Check sheet for the drawn part. Datum: minimum x, y, z corner. Units: mm. Give positions to 0.01 mm unless a question says otherwise; leave off trailing zeros. Loops run counter-clockwise (first coordinate to the right, second up) from the corner with the lowest first, then second, coordinate; pieces in that order, holes last. Notation, with made-up numbers: (20, 68) - (34, 68) arc R29 ccw to (34, 95) - close; hole circle Ø7 at (-16, 18.25). An arc over 180 degrees is marked (long way). One line per item, written item: value. Start each with the question number.
1. Sectioned sample at B-B (y = 39.5). Record the cut outline in (x, z), plus the area to 3 significant figures.
2. Sectioned sample at A-A (z = 7.5). Record the cut outline in (x, y).
3. Gauge pin test, flat end, axial feed: pin 1 (7.5 mm diameter, centred on y = 38.5, z = 8.5, fed in from -X). Record the tip position at first contact, or that the pin passes through.
4. Scan line: L1, parallel to X at y = 12.5, z = 6.25. Record every from-to range of solid material in increasing order. Write a range as [from, to].
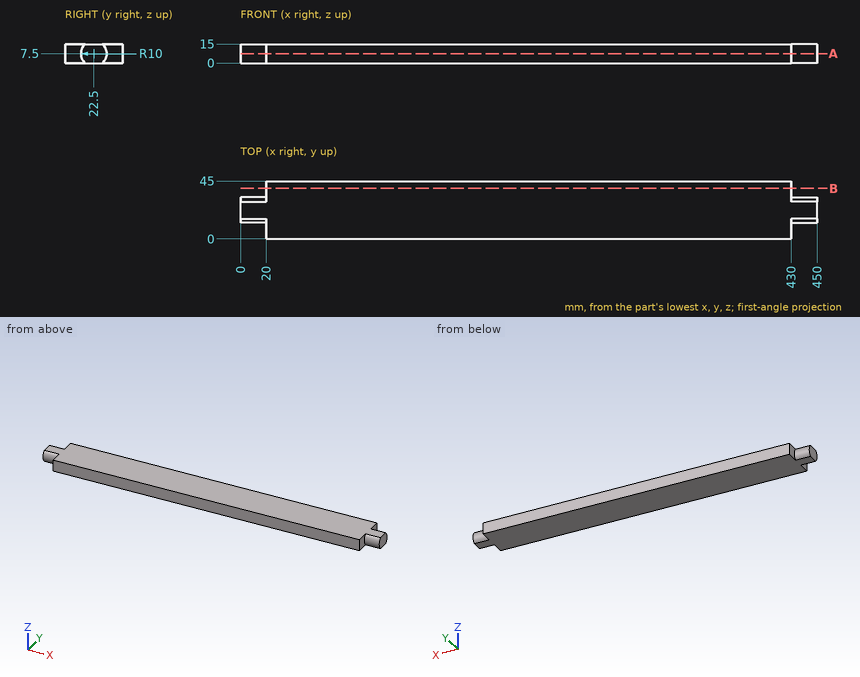
Results are:
1. outline: (20, 0) - (430, 0) - (430, 15) - (20, 15) - close
1. area: 6,150 mm^2
2. outline: (0, 12.5) - (20, 12.5) - (20, 0) - (430, 0) - (430, 12.5) - (450, 12.5) - (450, 32.5) - (430, 32.5) - (430, 45) - (20, 45) - (20, 32.5) - (0, 32.5) - close
3. pin 1: stops at x = 20
4. L1: x = [20, 430]
